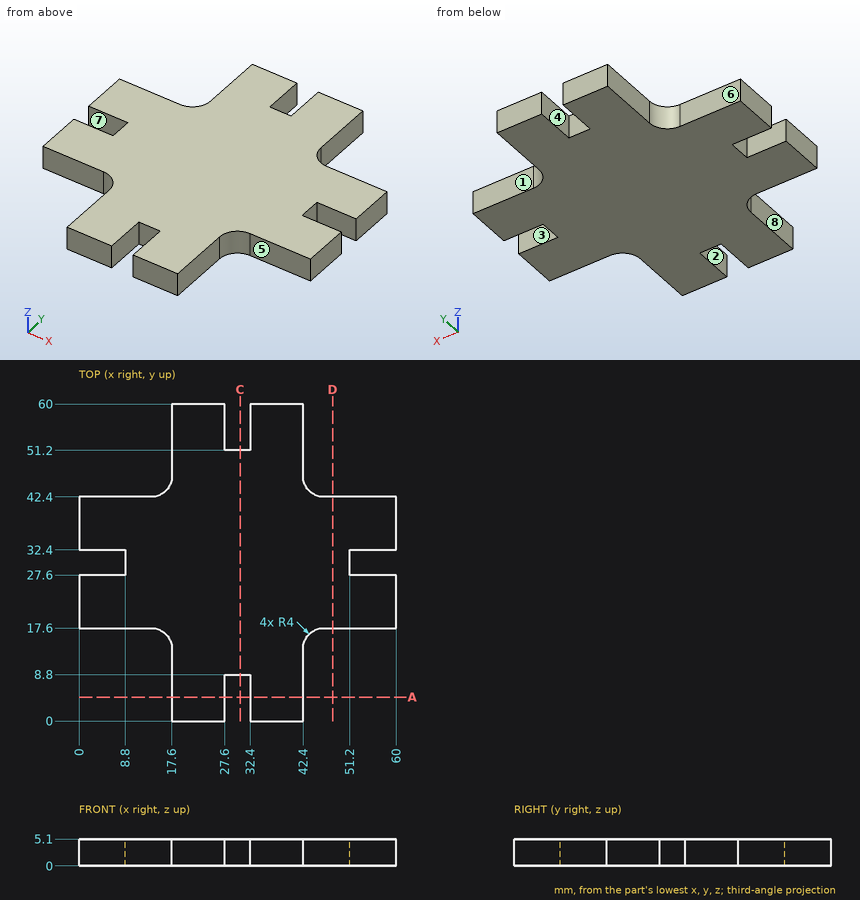
Design review of the part shown in the three views and the two pictorial views. Dimensions are in mm from the part's minimum x, y and z. A direction names the side the tool comes from. Coordinates: 2 decimals unless noted, no trailing zeros. Write each loop counter-clockwise with the first axis right and the second up, starting at its lowest first coordinate (ties: lowest second). Pieces come first, ordered by that corner, then holes. Notation, with made-up numbers: (49.5, 0) -> (89.5, 0) arc R11 ccw to (89.5, 14) -> close; hole circle Ø11 at (83, 54.25). An arc over 180 degrees is marked (long way). Answer in a Markdown table with one row per item.
1. Draft analysis for pull direction Y (two halves, no side actions). For the marked faces 5, 6, 7 and 8, state which applies: +Y half, -Y half, draft (parallel to the pull), parting line (faces both ways), or undercut.
Answers below:
| item | result |
|---|---|
| face 5 | -Y half |
| face 6 | +Y half |
| face 7 | undercut |
| face 8 | draft |
2. Wall thickness on probe 1 along X at (y, z) = (54.5, 2.5); probe 2 along Y at (x, z) = (48.5, 2.95); probe 3 along Y at (x, z) = (30, 0.7): over which ranges is each line inside the solid? List them lowest first. Write a range as [from, to].
Answers below:
| item | result |
|---|---|
| probe 1 | x = [17.6, 27.6], [32.4, 42.4] |
| probe 2 | y = [17.6, 42.4] |
| probe 3 | y = [8.8, 51.2] |
3. We need section A-A, the plane y = 4.5. State the section outline as (x, z) points, and give its area (3 significant figures).
Answers below:
| item | result |
|---|---|
| outline | (17.6, 0) -> (27.6, 0) -> (27.6, 5.1) -> (17.6, 5.1) -> close; (32.4, 0) -> (42.4, 0) -> (42.4, 5.1) -> (32.4, 5.1) -> close |
| area | 102 mm^2 |
4. We need section C-C, the plane x = 30.5. State the section outline as (y, z) points, and give its area (3 significant figures).
Answers below:
| item | result |
|---|---|
| outline | (8.8, 0) -> (51.2, 0) -> (51.2, 5.1) -> (8.8, 5.1) -> close |
| area | 216 mm^2 |
5. For the marked faces 1, 2, 3 and 4, list the 3-axis set-ups (+Z, -Z, +X, -X, +Y, -Y) from which the entire face can be reached by the end or side of a thin tool; tool diameter is ignored.
Answers below:
| item | result |
|---|---|
| face 1 | +Z, -Z, +X, +Y |
| face 2 | +Z, -Z, -Y |
| face 3 | +Z, -Z, +X |
| face 4 | +Z, -Z, +Y |
6. Clearance check with flat-ended pins moving along their axes: pin 1 Ø1.5 at (y, z) = (54.5, 2) entering from +X; pin 2 Ø2.5 at (y, z) = (29.5, 3.5) entering from +X; pin 3 Ø1.5 at (y, z) = (6, 2) entering from -X. State where each tip first meets the part, or that it passes through.
Answers below:
| item | result |
|---|---|
| pin 1 | stops at x = 42.4 |
| pin 2 | stops at x = 51.2 |
| pin 3 | stops at x = 17.6 |
7. We need section D-D, the plane x = 48. State the section outline as (y, z) points.
Answers below:
| item | result |
|---|---|
| outline | (17.6, 0) -> (42.4, 0) -> (42.4, 5.1) -> (17.6, 5.1) -> close |
